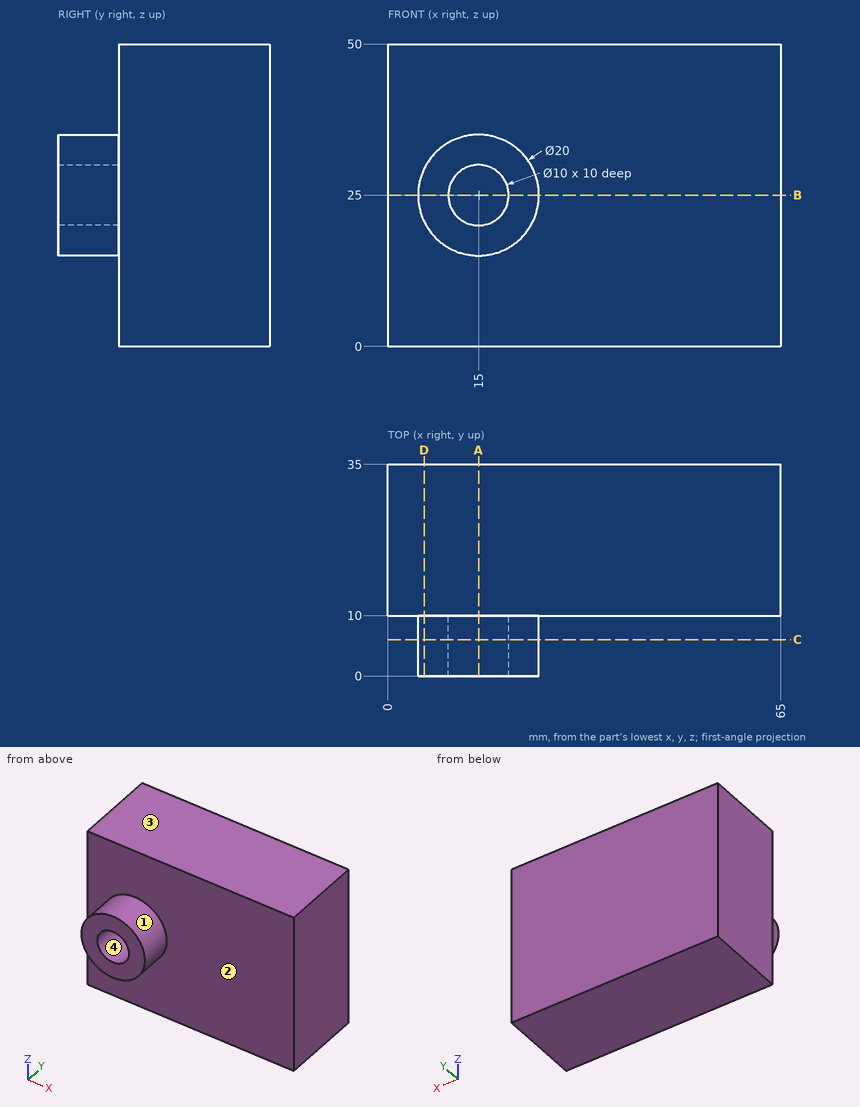
Answer from the drawing. Dimensions are ordinates in mm from the lowest x, y and z of the part. Coordinates: 2 decimals unless noted, no trailing zeros. Order: outer loops, then holes, each group sorted by start corner. A loop starts at its lowest first (then second) coordinate and runs counter-clockwise, first axis right, second up. Notation, with made-up numbers: (76, 18.5) - (98, 18.5) arc R16 ccw to (98, 22.5) - close; hole circle Ø10 at (20, 18). An arc over 180 degrees is marked (long way). Answer as a JSON object with one key per item and string values. Group by question number.
Item 1: Section C-C (y = 6) is taken. Give the vertices of the cut face in (x, z).
Item 2: Consider probe 1 along X at (y, z) = (6, 25); probe 2 along Y at (x, z) = (50, 39.5); probe 3 along Z at (x, y) = (12, 5.5). Determine where each line is inside the solid, lowest interval first. Write a range as from..to.
Item 3: Section A-A (x = 15) is taken. Give the vertices of the cut face in (y, z), plus the area to 3 significant figures.
Item 4: The mould has two halves that part along Z. Classify the marked faces 1, 2, 3 and 4: +Z half, -Z half, draft (parallel to the pull), parting line (faces both ways), or undercut.
Item 5: A flat-ended cylindrical pin translates along its axis: P1, Ø1, axis at x = 43, z = 21, coming from the -Y side. Find the tip coordinate at first contact, or state that the pin passes through.
Item 6: Section B-B (z = 25) is taken. Give the vertices of the cut face in (x, y), plus the area to 4 significant figures.
Item 7: Section D-D (x = 6) is taken. Give the vertices of the cut face in (y, z).
Results are:
{
 "1": {"outline": "circle Ø20 at (15, 25); hole circle Ø10 at (15, 25)"},
 "2": {"probe 1": "x = 5..10, 20..25", "probe 2": "y = 10..35", "probe 3": "z = 15.46..21, 29..34.54"},
 "3": {"outline": "(0, 15) - (10, 15) - (10, 0) - (35, 0) - (35, 50) - (10, 50) - (10, 35) - (0, 35) - (0, 30) - (10, 30) - (10, 20) - (0, 20) - close", "area": "1,350 mm^2"},
 "4": {"face 1": "parting line", "face 2": "draft", "face 3": "+Z half", "face 4": "undercut"},
 "5": {"P1": "stops at y = 10"},
 "6": {"outline": "(0, 10) - (5, 10) - (5, 0) - (10, 0) - (10, 10) - (20, 10) - (20, 0) - (25, 0) - (25, 10) - (65, 10) - (65, 35) - (0, 35) - close", "area": "1,725 mm^2"},
 "7": {"outline": "(0, 20.64) - (10, 20.64) - (10, 0) - (35, 0) - (35, 50) - (10, 50) - (10, 29.36) - (0, 29.36) - close"}
}
